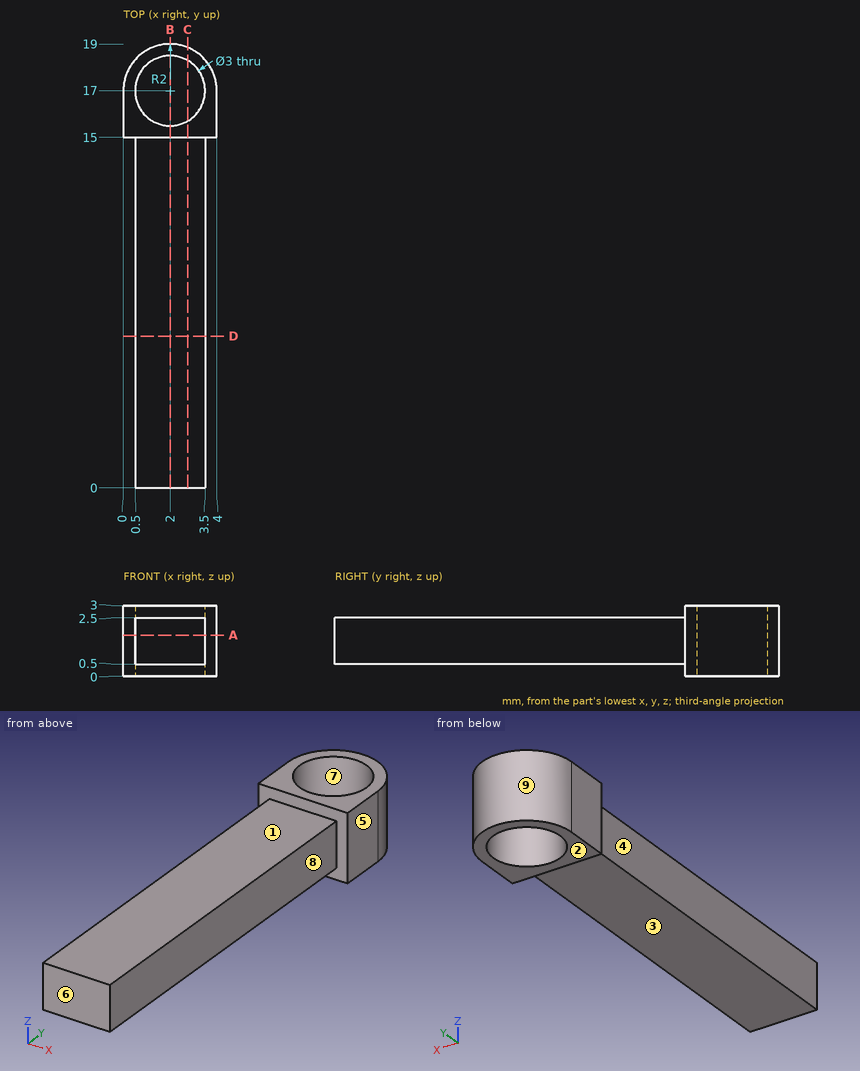
Job drawing, mm, ordinate dimensions from the low corner. One solid piece. A direction names the side the tool comes from. Round coordinates to 2 decimals unless told otherwise and drop trailing zeros. Order: outer loops, then holes, each group sorted by start corner. A loop starts at its lowest first (then second) coordinate and runs counter-clockwise, first axis right, second up. Notation, with made-up numbers: (26.5, -13.5) -> (71.5, -13.5) arc R21 cw to (71.5, 11.5) -> close; hole circle Ø1 at (34.25, 33.5). An arc over 180 degrees is marked (long way). Answer in a Markdown table with one row per item.
1) Band-saw the part on C-C on x = 2.75. Give the cut face in (y, z).
Values:
| item | result |
|---|---|
| outline | (0, 0.5) -> (15, 0.5) -> (15, 0) -> (15.7, 0) -> (15.7, 3) -> (15, 3) -> (15, 2.5) -> (0, 2.5) -> close; (18.3, 0) -> (18.85, 0) -> (18.85, 3) -> (18.3, 3) -> close |
2) Band-saw the part on D-D on y = 6.5. Give the cut face in (x, z).
Values:
| item | result |
|---|---|
| outline | (0.5, 0.5) -> (3.5, 0.5) -> (3.5, 2.5) -> (0.5, 2.5) -> close |
3) Band-saw the part on A-A on z = 1.75. Give the cut face in (x, y), and give its area (3 significant figures).
Values:
| item | result |
|---|---|
| outline | (0, 15) -> (0.5, 15) -> (0.5, 0) -> (3.5, 0) -> (3.5, 15) -> (4, 15) -> (4, 17) arc R2 ccw to (0, 17) -> close; hole circle Ø3 at (2, 17) |
| area | 52.2 mm2 |
4) Pin check, flat tips, straight feed: P1, Ø0.9, axis at x = 2.5, y = 7, coming from the +Z side; P2, Ø1, axis at y = 7, z = 2, coming from the +X side; P3, Ø0.9, axis at x = 1.5, y = 4.5, coming from the -Z side. Stop position of each tip, or through.
Values:
| item | result |
|---|---|
| P1 | z = 2.5 |
| P2 | x = 3.5 |
| P3 | z = 0.5 |
5) Mould opens along X. For the marked faces 6, 7, 8 and 9 say: released by +X, released by -X, zero draft, split by the parting line, or undercut.
Values:
| item | result |
|---|---|
| face 6 | zero draft |
| face 7 | undercut |
| face 8 | released by +X |
| face 9 | split by the parting line |
6) Band-saw the part on B-B on x = 2. Give the cut face in (y, z), and give its area (3 significant figures).
Values:
| item | result |
|---|---|
| outline | (0, 0.5) -> (15, 0.5) -> (15, 0) -> (15.5, 0) -> (15.5, 3) -> (15, 3) -> (15, 2.5) -> (0, 2.5) -> close; (18.5, 0) -> (19, 0) -> (19, 3) -> (18.5, 3) -> close |
| area | 33.0 mm2 |
7) Which spindle directions (+Z, -Z, +X, -X, +Y, -Y) get a long thin tool onto all of the face, cutting with end or side? Do the marked faces 1, 2, 3, 4 and 5. Say none if no direction does.
Values:
| item | result |
|---|---|
| face 1 | +Z, +X, -X, -Y |
| face 2 | -Z, +X, -X, +Y, -Y |
| face 3 | -Z, +X, -X, -Y |
| face 4 | +Z, -Z, -X, -Y |
| face 5 | +Z, -Z, +X, +Y, -Y |
8) Wall check: L1, parallel to Y at x = 2, z = 2.05; L2, parallel to Z at x = 1.2, y = 6.25; L3, parallel to X at y = 13.5, z = 1.95. Give the ranges that are in metal, low to high.
Values:
| item | result |
|---|---|
| L1 | 0 to 15.5, 18.5 to 19 |
| L2 | 0.5 to 2.5 |
| L3 | 0.5 to 3.5 |
